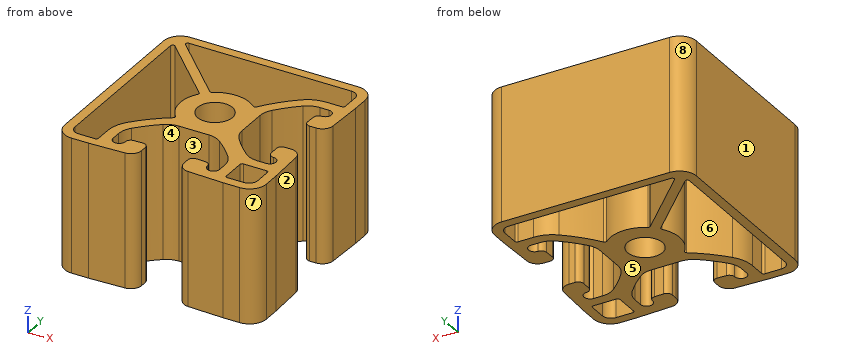
```python
from build123d import *

# Parameters (mm, degrees)
SKETCH1_R      = 3.302
EXTRUDE1_DEPTH = 25.4


with BuildPart() as part:
    # Sketch1 → Extrude1 (new body)
    with BuildSketch(Plane.XY):
        with BuildLine():
            Line((15.875, 19.05), (-15.875, 19.05))
            ThreePointArc((-15.875, 19.05), (-18.12006403, 18.12006403), (-19.05, 15.875))
            Line((-19.05, 15.875), (-19.05, -15.875))
            ThreePointArc((-19.05, -15.875), (-18.12006403, -18.12006403), (-15.875, -19.05))
            Line((-15.875, -19.05), (-12.7, -19.05))
            Line((-12.7, -19.05), (-5.954495972, -18.790863874))
            ThreePointArc((-5.954495972, -18.790863874), (-4.568340141, -18.169354143), (-4.0005, -16.760361628))
            Line((-4.0005, -16.760361628), (-4.0005, -15.552069001))
            ThreePointArc((-4.0005, -15.552069001), (-4.312003742, -14.819989072), (-5.055502014, -14.536817878))
            Line((-5.055502014, -14.536817878), (-6.782702014, -14.603170209))
            ThreePointArc((-6.782702014, -14.603170209), (-7.475165883, -14.913287543), (-7.759698458, -15.616651022))
            ThreePointArc((-7.759698458, -15.616651022), (-8.91004969, -16.763999564), (-10.0584, -15.614648356))
            Line((-10.0584, -15.614648356), (-10.0584, -13.931647412))
            ThreePointArc((-10.0584, -13.931647412), (-9.812696364, -12.53999053), (-9.105295238, -11.316608824))
            ThreePointArc((-9.105295238, -11.316608824), (-7.314841404, -9.397406099), (-5.335891418, -7.673219048))
            ThreePointArc((-5.335891418, -7.673219048), (-4.154656747, -7.029801128), (-2.828100791, -6.8072))
            Line((-2.828100791, -6.8072), (0, -6.8072))
            Line((0, -6.8072), (2.828100791, -6.8072))
            ThreePointArc((2.828100791, -6.8072), (4.154656747, -7.029801128), (5.335891418, -7.673219048))
            ThreePointArc((5.335891418, -7.673219048), (7.314841404, -9.397406099), (9.105295238, -11.316608824))
            ThreePointArc((9.105295238, -11.316608824), (9.812696364, -12.53999053), (10.0584, -13.931647412))
            Line((10.0584, -13.931647412), (10.0584, -15.614648356))
            ThreePointArc((10.0584, -15.614648356), (8.91004969, -16.763999564), (7.759698458, -15.616651022))
            ThreePointArc((7.759698458, -15.616651022), (7.475165883, -14.913287543), (6.782702014, -14.603170209))
            Line((6.782702014, -14.603170209), (5.055502014, -14.536817878))
            ThreePointArc((5.055502014, -14.536817878), (4.312003742, -14.819989072), (4.0005, -15.552069001))
            Line((4.0005, -15.552069001), (4.0005, -16.760361628))
            ThreePointArc((4.0005, -16.760361628), (4.568340141, -18.169354143), (5.954495972, -18.790863874))
            Line((5.954495972, -18.790863874), (12.7, -19.05))
            Line((12.7, -19.05), (15.875, -19.05))
            ThreePointArc((15.875, -19.05), (18.12006403, -18.12006403), (19.05, -15.875))
            Line((19.05, -15.875), (19.05, -12.7))
            Line((19.05, -12.7), (18.790863874, -5.954495972))
            ThreePointArc((18.790863874, -5.954495972), (18.169354143, -4.568340141), (16.760361628, -4.0005))
            Line((16.760361628, -4.0005), (15.552069001, -4.0005))
            ThreePointArc((15.552069001, -4.0005), (14.819989072, -4.312003742), (14.536817878, -5.055502014))
            Line((14.536817878, -5.055502014), (14.603170209, -6.782702014))
            ThreePointArc((14.603170209, -6.782702014), (14.913287543, -7.475165883), (15.616651022, -7.759698458))
            ThreePointArc((15.616651022, -7.759698458), (16.763999564, -8.91004969), (15.614648356, -10.0584))
            Line((15.614648356, -10.0584), (13.931647412, -10.0584))
            ThreePointArc((13.931647412, -10.0584), (12.53999053, -9.812696364), (11.316608824, -9.105295238))
            ThreePointArc((11.316608824, -9.105295238), (9.397406099, -7.314841404), (7.673219048, -5.335891418))
            ThreePointArc((7.673219048, -5.335891418), (7.029801128, -4.154656747), (6.8072, -2.828100791))
            Line((6.8072, -2.828100791), (6.8072, 0))
            Line((6.8072, 0), (6.8072, 2.828100791))
            ThreePointArc((6.8072, 2.828100791), (7.029801128, 4.154656747), (7.673219048, 5.335891418))
            ThreePointArc((7.673219048, 5.335891418), (9.397406099, 7.314841404), (11.316608824, 9.105295238))
            ThreePointArc((11.316608824, 9.105295238), (12.53999053, 9.812696364), (13.931647412, 10.0584))
            Line((13.931647412, 10.0584), (15.614648356, 10.0584))
            ThreePointArc((15.614648356, 10.0584), (16.763999564, 8.91004969), (15.616651022, 7.759698458))
            ThreePointArc((15.616651022, 7.759698458), (14.913287543, 7.475165883), (14.603170209, 6.782702014))
            Line((14.603170209, 6.782702014), (14.536817878, 5.055502014))
            ThreePointArc((14.536817878, 5.055502014), (14.819989072, 4.312003742), (15.552069001, 4.0005))
            Line((15.552069001, 4.0005), (16.760361628, 4.0005))
            ThreePointArc((16.760361628, 4.0005), (18.169354143, 4.568340141), (18.790863874, 5.954495972))
            Line((18.790863874, 5.954495972), (19.05, 12.7))
            Line((19.05, 12.7), (19.05, 15.875))
            ThreePointArc((19.05, 15.875), (18.12006403, 18.12006403), (15.875, 19.05))
        make_face()
        Circle(SKETCH1_R, mode=Mode.SUBTRACT)
        with BuildLine():
            Line((-4.191663684, 5.448899541), (-15.364356459, 16.621592316))
            ThreePointArc((-15.364356459, 16.621592316), (-15.446946878, 17.036802388), (-15.094948776, 17.272))
            Line((-15.094948776, 17.272), (15.621, 17.272))
            ThreePointArc((15.621, 17.272), (16.788433296, 16.788433296), (17.272, 15.621))
            Line((17.272, 15.621), (17.272, 12.4714))
            ThreePointArc((17.272, 12.4714), (17.160407684, 12.201992316), (16.891, 12.0904))
            Line((16.891, 12.0904), (13.931647412, 12.0904))
            ThreePointArc((13.931647412, 12.0904), (11.84416209, 11.721844546), (10.00908953, 10.660742857))
            ThreePointArc((10.00908953, 10.660742857), (7.259428949, 8.000870719), (4.906547928, 4.984332303))
            ThreePointArc((4.906547928, 4.984332303), (4.638901343, 4.819224111), (4.338293085, 4.91158257))
            ThreePointArc((4.338293085, 4.91158257), (0.40044901, 6.540953358), (-3.706747429, 5.40411452))
            ThreePointArc((-3.706747429, 5.40411452), (-3.957294594, 5.338921804), (-4.191663684, 5.448899541))
        make_face(mode=Mode.SUBTRACT)
        with BuildLine():
            Line((-5.448899541, 4.191663684), (-16.621592316, 15.364356459))
            ThreePointArc((-16.621592316, 15.364356459), (-17.036802388, 15.446946878), (-17.272, 15.094948776))
            Line((-17.272, 15.094948776), (-17.272, -15.621))
            ThreePointArc((-17.272, -15.621), (-16.788433296, -16.788433296), (-15.621, -17.272))
            Line((-15.621, -17.272), (-12.4714, -17.272))
            ThreePointArc((-12.4714, -17.272), (-12.201992316, -17.160407684), (-12.0904, -16.891))
            Line((-12.0904, -16.891), (-12.0904, -13.931647412))
            ThreePointArc((-12.0904, -13.931647412), (-11.721844546, -11.84416209), (-10.660742857, -10.00908953))
            ThreePointArc((-10.660742857, -10.00908953), (-8.000870719, -7.259428949), (-4.984332303, -4.906547928))
            ThreePointArc((-4.984332303, -4.906547928), (-4.819224111, -4.638901343), (-4.91158257, -4.338293085))
            ThreePointArc((-4.91158257, -4.338293085), (-6.540953358, -0.40044901), (-5.40411452, 3.706747429))
            ThreePointArc((-5.40411452, 3.706747429), (-5.338921804, 3.957294594), (-5.448899541, 4.191663684))
        make_face(mode=Mode.SUBTRACT)
        with BuildLine():
            Line((12.4714, -12.0904), (16.891, -12.0904))
            ThreePointArc((16.891, -12.0904), (17.160407684, -12.201992316), (17.272, -12.4714))
            Line((17.272, -12.4714), (17.272, -15.621))
            ThreePointArc((17.272, -15.621), (16.788433296, -16.788433296), (15.621, -17.272))
            Line((15.621, -17.272), (12.4714, -17.272))
            ThreePointArc((12.4714, -17.272), (12.201992316, -17.160407684), (12.0904, -16.891))
            Line((12.0904, -16.891), (12.0904, -12.4714))
            ThreePointArc((12.0904, -12.4714), (12.201992316, -12.201992316), (12.4714, -12.0904))
        make_face(mode=Mode.SUBTRACT)
    extrude(amount=EXTRUDE1_DEPTH)


solid = part.part
```
CAD build for the part. Positions are in the model's coordinates, mm. Face numbers are marked on the shaded views. A direction names the side the tool comes from. Give positions to 0.01 mm unless a question says otherwise; leave off trailing zeros. Loops run counter-clockwise (first coordinate to the right, second up) from the corner with the lowest first, then second, coordinate; pieces in that order, holes last. Notation, with made-up numbers: (24.5, 48) - (59.5, 48) arc R19 ccw to (59.5, 61) - close; hole circle Ø5 at (58.25, 68.25). An arc over 180 degrees is marked (long way). Put each result on its own line as item: value.
Q1. Tool access for the marked faces 1, 2, 3, 4 and 5: list every direction of +Z, -Z, +X, -X, +Y, -Y with a clear straight run to the whole face (end or side of a thin tool).
Filled in:
face 1: +Z, -Z, -X, +Y, -Y
face 2: +Z, -Z, +X
face 3: +Z, -Z, -Y
face 4: +Z, -Z
face 5: -Z, +X, -X, +Y, -Y
Q2. Slice it at A-A (x = 0). Give the cut face in (y, z).
Filled in:
outline: (-6.81, 0) - (-3.3, 0) - (-3.3, 25.4) - (-6.81, 25.4) - close; (3.3, 0) - (6.55, 0) - (6.55, 25.4) - (3.3, 25.4) - close; (17.27, 0) - (19.05, 0) - (19.05, 25.4) - (17.27, 25.4) - close
Q3. Mould opens along X. For the marked faces 6, 7 and 8 say: pulls with the +X half, pulls with the -X half, needs draft (parallel to the pull), parting line crosses it, or undercut.
Filled in:
face 6: undercut
face 7: pulls with the +X half
face 8: pulls with the -X half
Q4. Flat gauge pins, fed straight in: pin 1 (12 mm diameter, centred on x = 3, z = 13, fed in from -Y); pin 2 (3 mm diameter, centred on x = 1, z = 12, fed in from -Y); pin 3 (1 mm diameter, centred on x = 16.5, z = 8, fed in from -Y). Where does each tip first touch, or does it go through?
Filled in:
pin 1: stops at y = -18.91
pin 2: stops at y = -6.81
pin 3: stops at y = -19.05
Q5. Slice it at C-C (x = -8.5). Give the cut face in (y, z).
Filled in:
outline: (-18.89, 0) - (-16.69, 0) - (-16.69, 25.4) - (-18.89, 25.4) - close; (-10.62, 0) - (-7.72, 0) - (-7.72, 25.4) - (-10.62, 25.4) - close; (7.24, 0) - (9.76, 0) - (9.76, 25.4) - (7.24, 25.4) - close; (17.27, 0) - (19.05, 0) - (19.05, 25.4) - (17.27, 25.4) - close
Q6. Slice it at B-B (y = 1). Give the cut face in (x, z).
Filled in:
outline: (-19.05, 0) - (-17.27, 0) - (-17.27, 25.4) - (-19.05, 25.4) - close; (-6.48, 0) - (-3.15, 0) - (-3.15, 25.4) - (-6.48, 25.4) - close; (3.15, 0) - (6.81, 0) - (6.81, 25.4) - (3.15, 25.4) - close
Q7. Slice it at D-D (z = 22.25). Give the number of separate pieces and of enclosed holes in the cut face, plus the area to 3 significant figures.
Filled in:
separate pieces: 1
enclosed holes: 4
area: 515 mm²
Q8. Probe line 1 along Y through (x, z) = (0, 14.75); line 2 along X through (y, z) = (-10.5, 17); line 3 along X through (y, z) = (6, 14.5). List the from-to ranges inside material, lowest first.
Filled in:
line 1: y = -6.81 to -3.3, 3.3 to 6.55, 17.27 to 19.05
line 2: x = -19.05 to -17.27, -11.03 to -8.39, 8.39 to 18.97
line 3: x = -19.05 to -17.27, -7.26 to -4.74, -2.64 to 2.64, 5.62 to 8.21, 14.57 to 18.79
